Build history of the part. All positions in model axes, mm. A direction names the side the tool comes from. Coordinates: 2 decimals unless noted, no trailing zeros. One line per item, written item: value.
```python
from build123d import *

# Parameters (mm, degrees)
F1_DEPTH = 25.4


with BuildPart() as f1:
    # F0 (on Right) → F1 (new body)
    with BuildSketch(Plane.YZ):
        with BuildLine():
            Line((-33.02, -94.7882861604), (0, -94.7882861604))
            Line((0, -94.7882861604), (33.02, -94.7882861604))
            ThreePointArc((33.02, -94.7882861604), (36.6121024484, -96.276183712), (38.1, -99.8682861604))
            Line((38.1, -99.8682861604), (38.1, -113.8382861604))
            Line((38.1, -113.8382861604), (177.8, -113.8382861604))
            Line((177.8, -113.8382861604), (177.8, -99.8682861604))
            ThreePointArc((177.8, -99.8682861604), (179.2878975516, -96.276183712), (182.88, -94.7882861604))
            Line((182.88, -94.7882861604), (223.52, -94.7882861604))
            ThreePointArc((223.52, -94.7882861604), (227.1121024484, -96.276183712), (228.6, -99.8682861604))
            Line((228.6, -99.8682861604), (228.6, -113.8382861604))
            Line((228.6, -113.8382861604), (368.3, -113.8382861604))
            Line((368.3, -113.8382861604), (368.3, -99.8682861604))
            ThreePointArc((368.3, -99.8682861604), (369.7878975516, -96.276183712), (373.38, -94.7882861604))
            Line((373.38, -94.7882861604), (414.02, -94.7882861604))
            ThreePointArc((414.02, -94.7882861604), (417.6121024484, -96.276183712), (419.1, -99.8682861604))
            Line((419.1, -99.8682861604), (419.1, -113.8382861604))
            Line((419.1, -113.8382861604), (546.1, -113.8382861604))
            Line((546.1, -113.8382861604), (546.1, -99.8682861604))
            ThreePointArc((546.1, -99.8682861604), (547.5878975516, -96.276183712), (551.18, -94.7882861604))
            Line((551.18, -94.7882861604), (571.5, -94.7882861604))
            add(Edge.make_bspline(
                [(571.5, -94.7882861604), (572.9916402115, -51.8796445459), (572.0651404012, 35.9396927338), (525.960624218, 164.5377278328), (483.0139090485, 207.2824090719)],
                knots=[0, 0, 0, 0, 0.455226695, 1, 1, 1, 1], degree=3))
            Line((483.0139090485, 207.2824090719), (457.6139090485, 207.2824090719))
            ThreePointArc((457.6139090485, 207.2824090719), (454.4468485925, 215.6736583026), (457.6139090485, 224.0649075333))
            Line((457.6139090485, 224.0649075333), (457.6139090485, 234.5455965156))
            add(Edge.make_bspline(
                [(457.6139090485, 234.5455965156), (430.2923400603, 242.6197356959), (367.9016901724, 260.6701177346), (280.7948912625, 262.2175910558), (232.0806728363, 263.0830109119)],
                knots=[0.0166181854, 0.0166181854, 0.0166181854, 0.0166181854, 0.4500466426, 1, 1, 1, 1], degree=3))
            Line((232.0806728363, 263.0830109119), (232.0806728363, 209.2051863447))
            Line((232.0806728363, 209.2051863447), (377.5198757648, 186.3945573568))
            Line((377.5198757648, 186.3945573568), (483.9270131228, -5.2314990347))
            ThreePointArc((483.9270131228, -5.2314990347), (481.6642820093, -22.7701705112), (465.9854230078, -30.9493104209))
            Line((465.9854230078, -30.9493104209), (0, -30.9493104209))
            Line((0, -30.9493104209), (-465.9854230078, -30.9493104209))
            ThreePointArc((-465.9854230078, -30.9493104209), (-481.6642820093, -22.7701705112), (-483.9270131228, -5.2314990347))
            Line((-483.9270131228, -5.2314990347), (-377.5198757648, 186.3945573568))
            Line((-377.5198757648, 186.3945573568), (-232.0806728363, 209.2051863447))
            Line((-232.0806728363, 209.2051863447), (-232.0806728363, 263.0830109119))
            add(Edge.make_bspline(
                [(-457.6139090485, 234.5455965156), (-430.2923400603, 242.6197356959), (-367.9016901724, 260.6701177346), (-280.7948912625, 262.2175910558), (-232.0806728363, 263.0830109119)],
                knots=[0.0166181854, 0.0166181854, 0.0166181854, 0.0166181854, 0.4500466426, 1, 1, 1, 1], degree=3))
            Line((-457.6139090485, 234.5455965156), (-457.6139090485, 224.0649075333))
            ThreePointArc((-457.6139090485, 224.0649075333), (-454.4468485925, 215.6736583026), (-457.6139090485, 207.2824090719))
            Line((-457.6139090485, 207.2824090719), (-483.0139090485, 207.2824090719))
            add(Edge.make_bspline(
                [(-571.5, -94.7882861604), (-572.9916402115, -51.8796445459), (-572.0651404012, 35.9396927338), (-525.960624218, 164.5377278328), (-483.0139090485, 207.2824090719)],
                knots=[0, 0, 0, 0, 0.455226695, 1, 1, 1, 1], degree=3))
            Line((-571.5, -94.7882861604), (-551.18, -94.7882861604))
            ThreePointArc((-551.18, -94.7882861604), (-547.5878975516, -96.276183712), (-546.1, -99.8682861604))
            Line((-546.1, -99.8682861604), (-546.1, -113.8382861604))
            Line((-546.1, -113.8382861604), (-419.1, -113.8382861604))
            Line((-419.1, -113.8382861604), (-419.1, -99.8682861604))
            ThreePointArc((-419.1, -99.8682861604), (-417.6121024484, -96.276183712), (-414.02, -94.7882861604))
            Line((-414.02, -94.7882861604), (-373.38, -94.7882861604))
            ThreePointArc((-373.38, -94.7882861604), (-369.7878975516, -96.276183712), (-368.3, -99.8682861604))
            Line((-368.3, -99.8682861604), (-368.3, -113.8382861604))
            Line((-368.3, -113.8382861604), (-228.6, -113.8382861604))
            Line((-228.6, -113.8382861604), (-228.6, -99.8682861604))
            ThreePointArc((-228.6, -99.8682861604), (-227.1121024484, -96.276183712), (-223.52, -94.7882861604))
            Line((-223.52, -94.7882861604), (-182.88, -94.7882861604))
            ThreePointArc((-182.88, -94.7882861604), (-179.2878975516, -96.276183712), (-177.8, -99.8682861604))
            Line((-177.8, -99.8682861604), (-177.8, -113.8382861604))
            Line((-177.8, -113.8382861604), (-38.1, -113.8382861604))
            Line((-38.1, -113.8382861604), (-38.1, -99.8682861604))
            ThreePointArc((-38.1, -99.8682861604), (-36.6121024484, -96.276183712), (-33.02, -94.7882861604))
        make_face()
    extrude(amount=F1_DEPTH)


solid = f1.part
```
Item 1: Drop flat-ended pins along their axis: P1, Ø4, axis at x = 11.5, z = -110.5, coming from the -Y side; P2, Ø12.5, axis at x = 8, y = -187, coming from the +Z side; P3, Ø11.5, axis at x = 17, z = 229.5, coming from the +Y side. Give the stop position or say it passes through.
Check result:
P1: stops at y = -546.1
P2: stops at z = -30.95
P3: stops at y = 457.61
Item 2: Pull direction Y, two halves, no side cores. Call faces 5 (the face through (13, -483, -113.838)), 6 (the face through (13, 232.081, 237)): released by +Y, released by -Y, zero draft, split by the parting line, or undercut.
Check result:
face 5: zero draft
face 6: undercut
Item 3: Probe probe 1 along Z at (x, y) = (3, -29); probe 2 along Z at (x, y) = (21, -297); probe 3 along Y at (x, z) = (18.75, 114). List the from-to ranges inside material, lowest first. Write a range as from..to.
Check result:
probe 1: z = -94.79..-30.95
probe 2: z = -113.84..-30.95, 199.02..261.45
probe 3: y = -540.23..-417.72, 417.72..540.23
Item 4: Tool access for faces 1 (the face through (12.52, 481.81, -22.56)), 2 (the face through (13, -232.081, 236)), 3 (the face through (13, 0, -94.788)), 4 (the face through (13, -561, -94.788)): list every direction of +Z, -Z, +X, -X, +Y, -Y with a clear straight run to the whole face (end or side of a thin tool).
Check result:
face 1: +X, -X
face 2: +Z, +X, -X
face 3: -Z, +X, -X
face 4: -Z, +X, -X, -Y
